Verification items for the finished model (mm, model axes). A direction names the side the tool comes from. Round coordinates to 2 decimals unless told otherwise and drop trailing zeros. Order: outer loops, then holes, each group sorted by start corner. A loop starts at its lowest first (then second) coordinate and runs counter-clockwise, first axis right, second up. Notation, with made-up numbers: (0, 26) -> (22, 26) arc R27 cw to (22, 49) -> close; hole circle Ø10 at (3, -8). An arc over 180 degrees is marked (long way). Put each result on its own line as item: value.
```python
from build123d import *

# Parameters (mm, degrees)
BOSS_EXTRUDE1_DEPTH = 16
SKETCH2_R           = 1.5025
CUT_EXTRUDE1_DEPTH  = 6.005
SKETCH3_R           = 1.5
CUT_EXTRUDE2_DEPTH  = 6


with BuildPart() as part:
    # Sketch1 → Boss-Extrude1 (new body)
    with BuildSketch(Plane(origin=(0, 0, 0), x_dir=(1, 0, 0), z_dir=(0, 1, 0))):
        Polygon((2.5, 1.443375673), (0, 2.886751346), (-2.5, 1.443375673), (-2.5, -1.443375673), (0, -2.886751346), (2.5, -1.443375673), align=None)
    extrude(amount=BOSS_EXTRUDE1_DEPTH)

    # Sketch2 → Cut-Extrude1 (cut)
    with BuildSketch(Plane(origin=(0, 0, 0), x_dir=(1, 0, 0), z_dir=(0, 1, 0))):
        Circle(SKETCH2_R)
    extrude(amount=CUT_EXTRUDE1_DEPTH, mode=Mode.SUBTRACT)

    # Sketch3 → Cut-Extrude2 (cut)
    with BuildSketch(Plane(origin=(0, 16, 0), x_dir=(1, 0, 0), z_dir=(0, 1, 0))):
        Polygon((0, 2.886751346), (-2.5, 1.443375673), (-2.5, -1.443375673), (0, -2.886751346), (2.5, -1.443375673), (2.5, 1.443375673), align=None)
        Circle(SKETCH3_R, mode=Mode.SUBTRACT)
    extrude(amount=-CUT_EXTRUDE2_DEPTH, mode=Mode.SUBTRACT)


solid = part.part
```
Item 1: Release check for a two-part mould opening along Z. For faces 4 (the face through (-1.233, 4.93, -2.175)), 5 (the face through (0, 6.005, 0)), 6 (the face through (-1.15, 0, 1.24)) record: pulls with the +Z half, pulls with the -Z half, needs draft (parallel to the pull), parting line crosses it, or undercut.
Geometry check:
face 4: pulls with the -Z half
face 5: undercut
face 6: needs draft
Item 2: Depth check by flat-ended pin: pin 1 Ø1.5 at (x, z) = (0, -0.5) entering from -Y (3 decimals); pin 2 Ø2 at (x, y) = (-0.5, 3) entering from -Z. Enter the tip coordinate at first touch or a pass-through.
Geometry check:
pin 1: y = 6.005
pin 2: z = -2.89
Item 3: Sectioned sample at D-D, the plane z = 2.35. Record the boundary of the cut face in (x, y).
Geometry check:
outline: (-0.93, 0) -> (0.93, 0) -> (0.93, 10) -> (-0.93, 10) -> close
Item 4: Material ranges on line 1 along X through (y, z) = (2.5, 0); line 2 along Y through (x, z) = (-0.75, -0.95) (3 decimals); line 3 along Y through (x, z) = (-1.9, 0.65), recorded low to high.
Geometry check:
line 1: -2.5 to -1.5, 1.5 to 2.5
line 2: 6.005 to 16
line 3: 0 to 10
Item 5: Sectioned sample at C-C, the plane y = 14. Record the boundary of the cut face in (x, z).
Geometry check:
outline: circle Ø3 at (0, 0)
Item 6: Sectioned sample at B-B, the plane x = -1.25. Record the boundary of the cut face in (y, z) (3 decimals).
Geometry check:
outline: (0, -2.165) -> (10, -2.165) -> (10, -0.829) -> (16, -0.829) -> (16, 0.829) -> (10, 0.829) -> (10, 2.165) -> (0, 2.165) -> (0, 0.834) -> (6.005, 0.834) -> (6.005, -0.834) -> (0, -0.834) -> close
Item 7: Tool access check on faces 1 (the face through (-1.5, 13.04, -0.07)), 2 (the face through (0, 16, 0)), 3 (the face through (1.433, 2.96, -0.451)). Record the directions out of +Z, -Z, +X, -X, +Y, -Y that give a thin tool (end or side, any length) a straight path to the whole face; none if there is none.
Geometry check:
face 1: +Y
face 2: +Z, -Z, +X, -X, +Y
face 3: -Y
Item 8: Sectioned sample at A-A, the plane z = 0. Record the boundary of the cut face in (x, y) (1 decimal).
Geometry check:
outline: (-2.5, 0) -> (-1.5, 0) -> (-1.5, 6) -> (1.5, 6) -> (1.5, 0) -> (2.5, 0) -> (2.5, 10) -> (1.5, 10) -> (1.5, 16) -> (-1.5, 16) -> (-1.5, 10) -> (-2.5, 10) -> close
